from build123d import *

# Parameters (mm, degrees)
SKETCH_1_R                      = 3
EXTRUDE_1_DEPTH                 = 1
EXTRUDE_2_DEPTH                 = 1
EXTRUDE_2_DEPTH_BACK            = 1
FILLET_1_R                      = 1
SKETCH_3_R                      = 2
EXTRUDE_3_DEPTH                 = 6.4
EXTRUDE_4_DEPTH                 = 2
CHAMFER_1_SIZE                  = 0.5
CHAMFER_2_SIZE                  = 1
CUT_EXTRUDE_1_REACH             = 10.602
CUT_EXTRUDE_1_DIRECTION_2_REACH = 10.602


with BuildPart() as part:
    # 草图1 → 凸台-拉伸1 (new body)
    with BuildSketch(Plane(origin=(0, 0, 0), x_dir=(1, 0, 0), z_dir=(0, 1, 0))):
        with Locations(Location((0, 0, 0), (0, 0, 270))):
            Circle(SKETCH_1_R)
    extrude(amount=EXTRUDE_1_DEPTH)

    # 草图2 → 凸台-拉伸2 (add, two sides: drawn at the far end of the back side and taken through both)
    with BuildSketch(Plane.XY.offset(-EXTRUDE_2_DEPTH_BACK)):
        Polygon((-3.75, 7), (3.75, 7), (4, 1), (-4, 1), align=None)
    extrude(amount=EXTRUDE_2_DEPTH + EXTRUDE_2_DEPTH_BACK)

    # 圆角1
    fillet_1_edges = [part.edges().sort_by_distance(p)[0] for p in [
        (-3.75, 7, 0),
        (3.75, 7, 0),
    ]]
    fillet(fillet_1_edges, radius=FILLET_1_R)

    # 草图3 → 凸台-拉伸3 (add)
    with BuildSketch(Plane(origin=(0, 0, 0), x_dir=(-1, 0, 0), z_dir=(0, -1, 0))):
        with Locations(Location((0, 0, 0), (0, 0, 270))):
            Circle(SKETCH_3_R)
    extrude(amount=EXTRUDE_3_DEPTH)

    # 草图4 → 凸台-拉伸4 (add)
    with BuildSketch(Plane(origin=(0, -6.4, 0), x_dir=(-1, 0, 0), z_dir=(0, -1, 0))):
        with BuildLine():
            Line((2.598076211, -1.5), (-2.598076211, -1.5))
            ThreePointArc((-2.598076211, -1.5), (-3, 0), (-2.598076211, 1.5))
            Line((-2.598076211, 1.5), (2.598076211, 1.5))
            ThreePointArc((2.598076211, 1.5), (3, 0), (2.598076211, -1.5))
        make_face()
    extrude(amount=-EXTRUDE_4_DEPTH)

    # 倒角1
    chamfer_1_edges = [part.edges().sort_by_distance(p)[0] for p in [
        (3, -6.4, 0),
        (-3, -6.4, 0),
    ]]
    chamfer(chamfer_1_edges, length=CHAMFER_1_SIZE)

    # 倒角2
    chamfer_2_edges = [part.edges().sort_by_distance(p)[0] for p in [
        (3, -4.4, 0),
        (-3, -4.4, 0),
    ]]
    chamfer(chamfer_2_edges, length=CHAMFER_2_SIZE - 0.0001)  # a hair under: the kernel refuses the full size

    # 草图5 → 切除-拉伸1 (cut, up to next)
    with BuildSketch(Plane(origin=(0, 0, 0), x_dir=(0, 0, -1), z_dir=(1, 0, 0)), mode=Mode.PRIVATE) as cut_extrude_1_sk1:
        Polygon((2, -5.2), (1, -6.4), (2, -6.4), align=None)
    cut_extrude_1_tool1 = extrude(cut_extrude_1_sk1.sketch, amount=-CUT_EXTRUDE_1_REACH, mode=Mode.PRIVATE) & part.part
    # 草图5 → 切除-拉伸1 (cut, up to next)
    with BuildSketch(Plane(origin=(0, 0, 0), x_dir=(0, 0, -1), z_dir=(1, 0, 0)), mode=Mode.PRIVATE) as cut_extrude_1_sk2:
        Polygon((-2, -5.2), (-2, -6.4), (-1, -6.4), align=None)
    cut_extrude_1_tool2 = extrude(cut_extrude_1_sk2.sketch, amount=-CUT_EXTRUDE_1_REACH, mode=Mode.PRIVATE) & part.part
    add(cut_extrude_1_tool1.solids().sort_by_distance((0, -6, -1.666667))[0], mode=Mode.SUBTRACT)
    add(cut_extrude_1_tool2.solids().sort_by_distance((0, -6, 1.666667))[0], mode=Mode.SUBTRACT)

    # 草图5 → 切除-拉伸1 direction 2 (cut, up to next)
    with BuildSketch(Plane(origin=(0, 0, 0), x_dir=(0, 0, -1), z_dir=(1, 0, 0)), mode=Mode.PRIVATE) as cut_extrude_1_direction_2_sk1:
        Polygon((2, -5.2), (1, -6.4), (2, -6.4), align=None)
    cut_extrude_1_direction_2_tool1 = extrude(cut_extrude_1_direction_2_sk1.sketch, amount=CUT_EXTRUDE_1_DIRECTION_2_REACH, mode=Mode.PRIVATE) & part.part
    # 草图5 → 切除-拉伸1 direction 2 (cut, up to next)
    with BuildSketch(Plane(origin=(0, 0, 0), x_dir=(0, 0, -1), z_dir=(1, 0, 0)), mode=Mode.PRIVATE) as cut_extrude_1_direction_2_sk2:
        Polygon((-2, -5.2), (-2, -6.4), (-1, -6.4), align=None)
    cut_extrude_1_direction_2_tool2 = extrude(cut_extrude_1_direction_2_sk2.sketch, amount=CUT_EXTRUDE_1_DIRECTION_2_REACH, mode=Mode.PRIVATE) & part.part
    add(cut_extrude_1_direction_2_tool1.solids().sort_by_distance((0, -6, -1.666667))[0], mode=Mode.SUBTRACT)
    add(cut_extrude_1_direction_2_tool2.solids().sort_by_distance((0, -6, 1.666667))[0], mode=Mode.SUBTRACT)


solid = part.part
Design review of the part built by this model. Coordinates are the model's own, in mm. A direction names the side the tool comes from. Give positions to 0.01 mm unless a question says otherwise; leave off trailing zeros. Loops run counter-clockwise (first coordinate to the right, second up) from the corner with the lowest first, then second, coordinate; pieces in that order, holes last. Notation, with made-up numbers: M 34.25,1.25 L 39.25,1.25 A8 cw 39.25,7.25 Z; hole C -0.5,-13.75 d7. An arc over 180 degrees is marked long. One line per question, with ' | ' between items. Start each with the question number.
1. For faces 1 (the face through (0, 1, 2)), 2 (the face through (-1.8, -5.3, -1.5)), 3 (the face through (2.4, -4.8, 0)), 4 (the face through (1.8, -5.3, -1.5)), list the 3-axis set-ups (+Z, -Z, +X, -X, +Y, -Y) from which the entire face can be reached by the end or side of a thin tool; tool diameter is ignored.
2. To check wall thickness, follow L1, parallel to Z at x = 1.5, y = 5.25; L2, parallel to X at y = 6, z = 0.1; L3, parallel to Y at x = 0, z = -2.5. State the ranges of each line that lie inside material, in increasing order.
3. Add section A-A (x = 0). Write out the cut boundary in (y, z).
4. Insertion check: P1, Ø0.6, axis at x = -2, y = -5.5, coming from the +Z side; P2, Ø1, axis at x = -2, y = -5, coming from the -Z side; P3, Ø4, axis at x = 1, y = -3.5, coming from the +Z side. Each pin has a flat end and moves straight along its axis. Give the tip position at first contact, or say it passes through.
5. Add section C-C (z = 2.3). Write out the cut boundary in (x, y), plus the area to 3 significant figures.
6. Add section D-D (x = -3.5). Write out the cut boundary in (y, z) (3 decimals), plus the area to 3 significant figures.
7. Add section B-B (y = -1.25). Write out the cut boundary in (x, z).
Worked out:
1) face 1: +Z, +X, -X, +Y | face 2: -Z, -X, -Y | face 3: +X | face 4: -Z, +X, -Y
2) L1: z = -1 to 1 | L2: x = -3.79 to 3.79 | L3: y = 0 to 1
3) outline: M -6.4,-1 L -5.2,-2 L 0,-2 L 0,-3 L 1,-3 L 1,-1 L 7,-1 L 7,1 L 1,1 L 1,3 L 0,3 L 0,2 L -5.2,2 L -6.4,1 Z
4) P1: stops at z = 1.5 | P2: stops at z = -1.5 | P3: stops at z = 2
5) outline: M -1.93,0 L 1.93,0 L 1.93,1 L -1.93,1 Z | area: 3.85 mm²
6) outline: M 1,-1 L 6.705,-1 L 6.705,1 L 1,1 Z | area: 11.4 mm²
7) outline: C 0,0 d4
